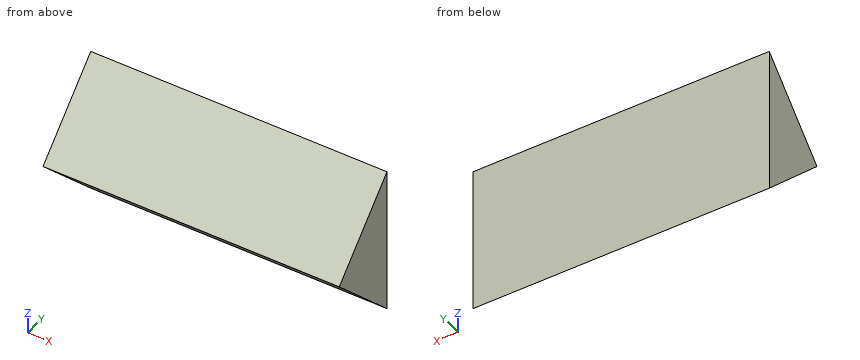
```python
from build123d import *

# Parameters (mm, degrees)
F0_W     = 101.6
F0_H     = 50.8
F1_DEPTH = 25.4
F4_DEPTH = 101.6
F5_DEPTH = 101.6


with BuildPart() as f1:
    # F0 (on Front) → F1 (new body)
    with BuildSketch(Plane.XZ):
        Rectangle(F0_W, F0_H)
    extrude(amount=F1_DEPTH)

    # F2 (on face) → F4 (cut)
    with BuildSketch(Plane.YZ.offset(50.8)):
        Polygon((-25.4, 25.4), (-25.4, 0), (0, 25.4), align=None)
    extrude(amount=-F4_DEPTH, mode=Mode.SUBTRACT)

    # F3 (on face) → F5 (cut)
    with BuildSketch(Plane(origin=(-50.8, 0, 0), x_dir=(0, -1, 0), z_dir=(-1, 0, 0))):
        Polygon((25.4, -25.4), (25.4, 0), (0, -25.4), align=None)
    extrude(amount=-F5_DEPTH, mode=Mode.SUBTRACT)


solid = f1.part
```
Geometry check sheet. Reference: the model listing, model coordinates, mm. Give positions to 0.01 mm unless a question says otherwise; leave off trailing zeros. Order: outer loops, then holes, each group sorted by start corner. A loop starts at its lowest first (then second) coordinate and runs counter-clockwise, first axis right, second up. Notation, with made-up numbers: (-36, 30) -> (9, 30) arc R23 ccw to (9, 47) -> close; hole circle Ø9 at (23, 84). An arc over 180 degrees is marked (long way). Write each question's results on one line, items separated by ' | '. Start each with the question number.
(1) Gauge pin test, flat ends, axial feed: P1, Ø1.5, axis at x = -37.5, y = -12.5, coming from the +Z side; P2, Ø12, axis at x = 11.5, y = -15, coming from the -Z side; P3, Ø5, axis at x = 24, z = 11.5, coming from the -Y side. Record the tip position at first contact, or that the pin passes through.
(2) Sectioned sample at A-A (z = 17). Enter the section's corners in (x, y), plus the area to 3 significant figures.
(3) Scan lines: line 1 (Y direction, x = 42.5, z = -15.5); line 2 (Z direction, x = -44, y = -8); line 3 (Z direction, x = 33, y = -10.25). Record each from-to range of solid material in increasing order.
(4) Sectioned sample at C-C (x = 5.5). Enter the section's corners in (y, z), plus the area to 3 significant figures.
(5) Sectioned sample at B-B (y = -15). Enter the section's corners in (x, z), plus the area to 3 significant figures.
Answer below:
1) P1: z = 13.65 | P2: z = -16.4 | P3: y = -16.4
2) outline: (-50.8, -8.4) -> (50.8, -8.4) -> (50.8, 0) -> (-50.8, 0) -> close | area: 853 mm2
3) line 1: -9.9 to 0 | line 2: -17.4 to 17.4 | line 3: -15.15 to 15.15
4) outline: (-25.4, 0) -> (0, -25.4) -> (0, 25.4) -> close | area: 645 mm2
5) outline: (-50.8, -10.4) -> (50.8, -10.4) -> (50.8, 10.4) -> (-50.8, 10.4) -> close | area: 2,110 mm2
